Verification items for the finished model (mm, model axes). A direction names the side the tool comes from. Give positions to 0.01 mm unless a question says otherwise; leave off trailing zeros. Order: outer loops, then holes, each group sorted by start corner. A loop starts at its lowest first (then second) coordinate and runs counter-clockwise, first axis right, second up. Notation, with made-up numbers: M 36,16.25 L 87,16.25 A32 cw 87,47.25 Z; hole C 17,-3 d1. An arc over 180 degrees is marked long. Answer as a JSON object with one key per item and string values.
```python
from build123d import *

# Parameters (mm, degrees)
SKETCH1_W           = 94.999999992
SKETCH1_H           = 162.000000104
BOSS_EXTRUDE1_DEPTH = 30
SKETCH2_W           = 90.000000086
SKETCH2_H           = 156.999999944
CUT_EXTRUDE1_DEPTH  = 30
SKETCH3_W           = 13
SKETCH3_H           = 2
BOSS_EXTRUDE2_DEPTH = 2.314
SKETCH4_W           = 13
SKETCH4_H           = 2
CUT_EXTRUDE2_DEPTH  = 6.632
CUT_EXTRUDE3_START  = -6.632
CUT_EXTRUDE3_DEPTH  = 6.632
CUT_EXTRUDE4_DEPTH  = 6.632
BOSS_EXTRUDE3_DEPTH = 2.54


with BuildPart() as part:
    # Sketch1 → Boss-Extrude1 (new body)
    with BuildSketch(Plane(origin=(0, 0, 0), x_dir=(1, 0, 0), z_dir=(0, 1, 0))):
        Rectangle(SKETCH1_W, SKETCH1_H)
    extrude(amount=BOSS_EXTRUDE1_DEPTH)

    # Sketch2 → Cut-Extrude1 (cut)
    with BuildSketch(Plane(origin=(0, 30, 0), x_dir=(1, 0, 0), z_dir=(0, 1, 0))):
        Rectangle(SKETCH2_W, SKETCH2_H)
    extrude(amount=-CUT_EXTRUDE1_DEPTH, mode=Mode.SUBTRACT)

    # Sketch3 → Boss-Extrude2 (add)
    with BuildSketch(Plane(origin=(47.499999996, 0, 0), x_dir=(0, 0, -1), z_dir=(1, 0, 0))):
        with BuildLine():
            Line((71.695000052, 12.46), (62.805000052, 12.46))
            ThreePointArc((62.805000052, 12.46), (60.265000052, 15), (62.805000052, 17.54))
            Line((62.805000052, 17.54), (71.695000052, 17.54))
            ThreePointArc((71.695000052, 17.54), (74.235000052, 15), (71.695000052, 12.46))
        make_face()
        with BuildLine():
            Line((53.744999952, 12.46), (44.854999952, 12.46))
            ThreePointArc((44.854999952, 12.46), (42.314999952, 15), (44.854999952, 17.54))
            Line((44.854999952, 17.54), (53.744999952, 17.54))
            ThreePointArc((53.744999952, 17.54), (56.284999952, 15), (53.744999952, 12.46))
        make_face()
        with Locations((32.000000052, 15)):
            Rectangle(SKETCH3_W, SKETCH3_H)
        with BuildLine():
            Line((-37.609999928, 13.72000002), (-43.389999968, 13.72000002))
            ThreePointArc((-43.389999968, 13.72000002), (-44.669999948, 15), (-43.389999968, 16.27999998))
            Line((-43.389999968, 16.27999998), (-37.609999928, 16.27999998))
            ThreePointArc((-37.609999928, 16.27999998), (-36.329999948, 15), (-37.609999928, 13.72000002))
        make_face()
    extrude(amount=BOSS_EXTRUDE2_DEPTH)

    # Sketch4 → Cut-Extrude2 (cut)
    with BuildSketch(Plane(origin=(49.813999996, 0, 0), x_dir=(0, 0, -1), z_dir=(1, 0, 0))):
        with Locations((32.000000052, 15)):
            Rectangle(SKETCH4_W, SKETCH4_H)
    extrude(amount=-CUT_EXTRUDE2_DEPTH, mode=Mode.SUBTRACT)

    # Sketch5 → Cut-Extrude3 (cut)
    with BuildSketch(Plane(origin=(49.813999996, 0, 0), x_dir=(0, 0, -1), z_dir=(1, 0, 0)).offset(CUT_EXTRUDE3_START)):
        with BuildLine():
            Line((-43.389999968, 16.27999998), (-37.609999928, 16.27999998))
            ThreePointArc((-37.609999928, 16.27999998), (-36.704903262, 15.905096666), (-36.329999948, 15))
            ThreePointArc((-36.329999948, 15), (-36.704903262, 14.094903334), (-37.609999928, 13.72000002))
            Line((-37.609999928, 13.72000002), (-43.389999968, 13.72000002))
            ThreePointArc((-43.389999968, 13.72000002), (-44.295096634, 14.094903334), (-44.669999948, 15))
            ThreePointArc((-44.669999948, 15), (-44.295096634, 15.905096666), (-43.389999968, 16.27999998))
        make_face()
    extrude(amount=CUT_EXTRUDE3_DEPTH, mode=Mode.SUBTRACT)

    # Sketch6 → Cut-Extrude4 (cut)
    with BuildSketch(Plane.ZY.offset(47.499999996)):
        with BuildLine():
            Line((-8.890000094, 16.28), (-3.11000001, 16.28))
            ThreePointArc((-3.11000001, 16.28), (-1.83000001, 15), (-3.11000001, 13.72))
            Line((-3.11000001, 13.72), (-8.890000094, 13.72))
            ThreePointArc((-8.890000094, 13.72), (-10.170000094, 15), (-8.890000094, 16.28))
        make_face()
    extrude(amount=-CUT_EXTRUDE4_DEPTH, mode=Mode.SUBTRACT)

    # Sketch9 → Boss-Extrude3 (add)
    with BuildSketch(Plane.ZY.offset(47.499999996)):
        with BuildLine():
            Line((-59.880000052, 9.717636473), (-67.500000052, 9.717636473))
            ThreePointArc((-67.500000052, 9.717636473), (-70.040000052, 12.257636473), (-67.500000052, 14.797636473))
            Line((-67.500000052, 14.797636473), (-59.880000052, 14.797636473))
            ThreePointArc((-59.880000052, 14.797636473), (-57.340000052, 12.257636473), (-59.880000052, 9.717636473))
        make_face()
    extrude(amount=BOSS_EXTRUDE3_DEPTH)


solid = part.part
```
Q1. Section check A-A on z = 59. Record the cut outline in (x, y).
Resolved:
{"outline": "M -47.5,0 L -45,0 L -45,30 L -47.5,30 Z; M 45,0 L 47.5,0 L 47.5,30 L 45,30 Z"}
Q2. Section check B-B on x = 12.5. Record the cut outline in (y, z).
Resolved:
{"outline": "M 0,-81 L 30,-81 L 30,-78.5 L 0,-78.5 Z; M 0,78.5 L 30,78.5 L 30,81 L 0,81 Z"}
Q3. Tool access check on faces 4 (the face through (49.814, 15, -49)), 5 (the face through (45, 15, 1)). Record the directions out of +Z, -Z, +X, -X, +Y, -Y that give a thin tool (end or side, any length) a straight path to the whole face; none if there is none.
Resolved:
{"face 4": "+Z, -Z, +X, +Y, -Y", "face 5": "+Y, -Y"}
Q4. Release check for a two-part mould opening along X. For faces 1 (the face through (49.814, 15, -67)), 2 (the face through (-1, 15, -78.5)), 3 (the face through (-50.04, 12, -64)) record: +X half, -X half, draft (parallel to the pull), parting line (faces both ways), or undercut.
Resolved:
{"face 1": "+X half", "face 2": "undercut", "face 3": "-X half"}
Q5. Material ranges on L1, parallel to X at y = 16.25, z = 74.5; L2, parallel to Z at x = -39.5, y = 10.25, recorded low to high.
Resolved:
{"L1": "x = -47.5 to -45, 45 to 47.5", "L2": "z = -81 to -78.5, 78.5 to 81"}
Q6. Section check C-C on y = 7. Record the cut outline in (x, z).
Resolved:
{"outline": "M -47.5,-81 L 47.5,-81 L 47.5,81 L -47.5,81 Z; hole M -45,-78.5 L 45,-78.5 L 45,78.5 L -45,78.5 Z"}
Q7. Gauge pin test, flat ends, axial feed: pin 1 Ø15 at (y, z) = (10, 23) entering from +X; pin 2 Ø1.9 at (x, z) = (48.5, -51) entering from +Y; pin 3 Ø9 at (y, z) = (18.5, -40) entering from -X. Record the tip position at first contact, or that the pin passes through.
Resolved:
{"pin 1": "stops at x = 47.5", "pin 2": "stops at y = 17.54", "pin 3": "stops at x = -47.5"}
